CAD build for the part. Positions are in the model's coordinates, mm. Face numbers are marked on the shaded views. Give positions to 0.01 mm unless a question says otherwise; leave off trailing zeros. Order: outer loops, then holes, each group sorted by start corner. A loop starts at its lowest first (then second) coordinate and runs counter-clockwise, first axis right, second up. Notation, with made-up numbers: (-10.5, 45.25) -> (41.5, 45.25) arc R25 ccw to (41.5, 74.25) -> close; hole circle Ø8 at (73.25, -12). An arc over 180 degrees is marked (long way). Use one line per item in the form item = value. Start each with the question number.
1) Cut at C-C, the plane x = -8.5. Give the cut face in (y, z), and give its area (3 significant figures).
2) Drop flat-ended pins along their axis: P1, Ø8, axis at x = 22.5, z = -19.5, coming from the -Y side; P2, Ø6, axis at x = 21.73, z = -20, coming from the -Y side; P3, Ø3, axis at x = -18.5, y = -28, coming from the -Z side. Give the stop position or say it passes through.
3) Cut at A-A, the plane z = 0. Give the cut face in (x, y).
4) Cut at B-B, the plane x = 0. Give the cut face in (y, z), and give its area (3 significant figures).
5) Probe line 1 (Z direction, x = 0, y = 4); line 2 (Z direction, x = -2, y = -21); line 3 (X direction, y = -7.5, z = -0.5). List the from-to ranges inside material, lowest first.
6) Cut at D-D, the plane z = 8. Give the cut face in (x, y).
7) Mould opens along Z. For the marked faces 1, 2 and 3 say: pulls with the +Z half, pulls with the -Z half, needs draft (parallel to the pull), parting line crosses it, or undercut.
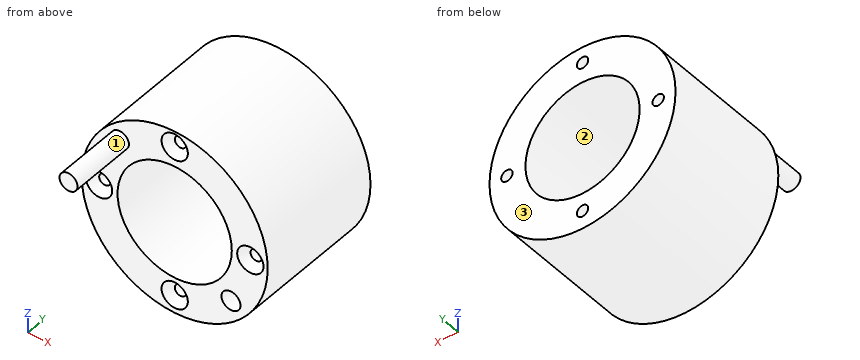
from build123d import *

# Parameters (mm, degrees)
F0_R           = 35.917539
F0_R_2         = 22.055201
F1_DEPTH       = 25.4
F3_D           = 4.4
F3_CSINK_D     = 10.16
F3_CSINK_ANGLE = 90
F4_R           = 3.4798
F5_DEPTH       = 25.4
F6_R           = 3.685712
F7_DEPTH       = 25.4


with BuildPart() as f1:
    # F0 (on Front) → F1 (new body, symmetric)
    with BuildSketch(Plane.XZ):
        Circle(F0_R)
        Circle(F0_R_2, mode=Mode.SUBTRACT)
    extrude(amount=F1_DEPTH, both=True)

    # F3 (through all)
    with Locations(Plane.XZ.offset(25.4)):
        with Locations((-29.212285, 0), (0, 29.787894), (29.212283, 0), (0, -28.924478)):
            CounterSinkHole(F3_D / 2, F3_CSINK_D / 2, counter_sink_angle=F3_CSINK_ANGLE)

    # F4 (on face) → F5 (join)
    with BuildSketch(Plane.XZ.offset(25.4)):
        with Locations((-21.153724, 21.729333)):
            Circle(F4_R)
    extrude(amount=F5_DEPTH)

    # F6 (on face) → F7 (cut)
    with BuildSketch(Plane.XZ.offset(25.4)):
        with Locations((21.729335, -20.002501)):
            Circle(F6_R)
    extrude(amount=-F7_DEPTH, mode=Mode.SUBTRACT)


solid = f1.part
Result:
q1.outline = (-25.4, -34.9) -> (25.4, -34.9) -> (25.4, -20.35) -> (-25.4, -20.35) -> close; (-25.4, 20.35) -> (25.4, 20.35) -> (25.4, 34.9) -> (-25.4, 34.9) -> close
q1.area = 1,480 mm²
q2.P1 = -25.4
q2.P2 = 0
q2.P3 = 18.45
q3.outline = (-35.92, -25.4) -> (-34.29, -25.4) -> (-31.41, -22.52) -> (-31.41, 25.4) -> (-35.92, 25.4) -> close; (-27.01, -22.52) -> (-24.13, -25.4) -> (-22.06, -25.4) -> (-22.06, 25.4) -> (-27.01, 25.4) -> close; (22.06, -25.4) -> (24.13, -25.4) -> (27.01, -22.52) -> (27.01, 25.4) -> (22.06, 25.4) -> close; (31.41, -22.52) -> (34.29, -25.4) -> (35.92, -25.4) -> (35.92, 25.4) -> (31.41, 25.4) -> close
q4.outline = (-25.4, -35.92) -> (25.4, -35.92) -> (25.4, -31.12) -> (-22.52, -31.12) -> (-25.4, -34) -> close; (-25.4, -23.84) -> (-22.52, -26.72) -> (25.4, -26.72) -> (25.4, -22.06) -> (-25.4, -22.06) -> close; (-25.4, 22.06) -> (25.4, 22.06) -> (25.4, 27.59) -> (-22.52, 27.59) -> (-25.4, 24.71) -> close; (-25.4, 34.87) -> (-22.52, 31.99) -> (25.4, 31.99) -> (25.4, 35.92) -> (-25.4, 35.92) -> close
q4.area = 945 mm²
q5.line_1 = -35.92 to -31.12, -26.72 to -22.06, 22.06 to 27.59, 31.99 to 35.92
q5.line_2 = -35.86 to -29.84, -28.01 to -21.96, 21.96 to 28.87, 30.7 to 35.86
q5.line_3 = -35.91 to -31.35, -27.07 to -22.05, 22.05 to 27.07, 31.35 to 35.91
q6.outline = (-35.02, -25.4) -> (-20.55, -25.4) -> (-20.55, 25.4) -> (-35.02, 25.4) -> close; (20.55, -25.4) -> (35.02, -25.4) -> (35.02, 25.4) -> (20.55, 25.4) -> close
q7.face_1 = parting line crosses it
q7.face_2 = undercut
q7.face_3 = needs draft
